from build123d import *

# Parameters (mm, degrees)
BOSS_EXTRUDE1_DEPTH = 22
SKETCH2_R           = 3.75
CUT_EXTRUDE1_DEPTH  = 5
SKETCH3_R           = 2.4
CUT_EXTRUDE2_DEPTH  = 5
SKETCH4_R           = 3.75
CUT_EXTRUDE3_DEPTH  = 5
SKETCH5_R           = 2.4
CUT_EXTRUDE4_DEPTH  = 5


with BuildPart() as part:
    # Sketch1 → Boss-Extrude1 (new body)
    with BuildSketch(Plane(origin=(0, 0, 0), x_dir=(0, 0, -1), z_dir=(1, 0, 0))):
        Polygon((0, 0), (-12, 0), (-12, -8), (8, -8), (8, 12), (0, 12), align=None)
    extrude(amount=BOSS_EXTRUDE1_DEPTH)

    # Sketch2 → Cut-Extrude1 (cut)
    with BuildSketch(Plane.XY):
        with Locations((11, 6)):
            Circle(SKETCH2_R)
    extrude(amount=-CUT_EXTRUDE1_DEPTH, mode=Mode.SUBTRACT)

    # Sketch3 → Cut-Extrude2 (cut)
    with BuildSketch(Plane.XY.offset(-5)):
        with Locations((11, 6)):
            Circle(SKETCH3_R)
    extrude(amount=-CUT_EXTRUDE2_DEPTH, mode=Mode.SUBTRACT)

    # Sketch4 → Cut-Extrude3 (cut)
    with BuildSketch(Plane(origin=(0, 0, 0), x_dir=(1, 0, 0), z_dir=(0, 1, 0))):
        with Locations(Location((11, -6, 0), (0, 0, 270))):
            Circle(SKETCH4_R)
    extrude(amount=-CUT_EXTRUDE3_DEPTH, mode=Mode.SUBTRACT)

    # Sketch5 → Cut-Extrude4 (cut)
    with BuildSketch(Plane(origin=(0, -5, 0), x_dir=(1, 0, 0), z_dir=(0, 1, 0))):
        with Locations(Location((11, -6, 0), (0, 0, 270))):
            Circle(SKETCH5_R)
    extrude(amount=-CUT_EXTRUDE4_DEPTH, mode=Mode.SUBTRACT)


solid = part.part
The model under review builds one solid part; all positions refer to its coordinate system, in mm. A direction names the side the tool comes from. Coordinates: 2 decimals unless noted, no trailing zeros. Write each loop counter-clockwise with the first axis right and the second up, starting at its lowest first coordinate (ties: lowest second). Pieces come first, ordered by that corner, then holes. Notation, with made-up numbers: (38.5, 80) - (54.5, 80) arc R19 cw to (54.5, 94) - close; hole circle Ø9 at (57.5, -32.75). An arc over 180 degrees is marked (long way). Answer as a JSON object with one key per item and string values. Group by question number.
1. Add section D-D (z = -1). Give the boundary of the cut face in (x, y), plus the area to 3 significant figures.
2. Clearance check with flat-ended pins moving along their axes: pin 1 Ø1.5 at (x, y) = (10.5, 1) entering from +Z; pin 2 Ø4 at (x, z) = (12.5, 5) entering from +Y. State where each tip first meets the part, or that it passes through.
3. Mouldability with a two-part tool opening along X and no side actions: class faces 1 (the face through (0, -2, 0)), 2 (the face through (13.45, 5.22, -5)), 3 (the face through (8, 9, 0)) as pulls with the +X half, pulls with the -X half, needs draft (parallel to the pull), parting line crosses it, or undercut.
4. Add section A-A (x = 11). Give the boundary of the cut face in (y, z), plus the area to 3 significant figures.
5. To check wall thickness, follow probe 1 along X at (y, z) = (-2.55, 6); probe 2 along Y at (x, z) = (11, -6.55); probe 3 along Y at (x, z) = (11, -3). State the ranges of each line that lie inside material, in increasing order.
6. Machinability: for faces 4 (the face through (10.22, -5, 8.45)), 5 (the face through (11, 12, -4)), 6 (the face through (8.024, 3.718, -2.465)), 7 (the face through (8, 0, 3)), 8 (the face through (11, 2, -8)), which of the approach directions +Z, -Z, +X, -X, +Y, -Y give a long, thin tool a straight path to every point of the face, cutting with its end or side? Answer none if there is none.
7. Add section B-B (z = 6). Give the boundary of the cut face in (x, y), plus the area to 3 significant figures.
Findings:
{
 "1": {"outline": "(0, -8) - (22, -8) - (22, 12) - (0, 12) - close; hole circle Ø7.5 at (11, 6)", "area": "396 mm²"},
 "2": {"pin 1": "z = 0", "pin 2": "y = 0"},
 "3": {"face 1": "pulls with the -X half", "face 2": "undercut", "face 3": "needs draft"},
 "4": {"outline": "(-8, -8) - (3.6, -8) - (3.6, -5) - (2.25, -5) - (2.25, 0) - (0, 0) - (0, 2.25) - (-5, 2.25) - (-5, 3.6) - (-8, 3.6) - close; (-8, 8.4) - (-5, 8.4) - (-5, 9.75) - (0, 9.75) - (0, 12) - (-8, 12) - close; (8.4, -8) - (12, -8) - (12, 0) - (9.75, 0) - (9.75, -5) - (8.4, -5) - close", "area": "152 mm²"},
 "5": {"probe 1": "0 to 7.25, 14.75 to 22", "probe 2": "-8 to 3.6, 8.4 to 12", "probe 3": "-8 to 2.25, 9.75 to 12"},
 "6": {"face 4": "+Y", "face 5": "+Z, -Z, +X, -X, +Y", "face 6": "+Z", "face 7": "+Z, +X, -X, +Y", "face 8": "-Z, +X, -X, +Y, -Y"},
 "7": {"outline": "(0, -8) - (8.6, -8) - (8.6, -5) - (7.25, -5) - (7.25, 0) - (0, 0) - close; (13.4, -8) - (22, -8) - (22, 0) - (14.75, 0) - (14.75, -5) - (13.4, -5) - close", "area": "124 mm²"}
}
